Geometry check sheet. Reference: the model listing, model coordinates, mm. A direction names the side the tool comes from. Coordinates: 2 decimals unless noted, no trailing zeros. Loops run counter-clockwise (first coordinate to the right, second up) from the corner with the lowest first, then second, coordinate; pieces in that order, holes last.
Autodesk Inventor part; units mm, degrees
ref_plane "YZ Plane" through (0, 0, 0) normal (1, 0, 0) x (0, 1, 0)
ref_plane "XZ Plane" through (0, 0, 0) normal (0, 1, 0) x (-1, 0, 0)
ref_plane "XY Plane" through (0, 0, 0) normal (0, 0, 1) x (1, 0, 0)
sketch "Sketch1" plane through (0, 0, 0) normal (0, 0, 1) x (1, 0, 0)
  line L0 (0, 0) -> (25.4, 0)
  line L1 (25.4, 0) -> (25.4, 50.8)
  line L2 (25.4, 50.8) -> (0, 50.8)
  line L3 (0, 50.8) -> (0, 0)
  dimension "d0" = 25.4
  dimension "d1" = 50.8
extrude "Extrusion1" add sketch "Sketch1" along normal blind 254
shell "Shell1" thickness 2.54 removed faces 2 at (8.4667, 33.8667, 0) at (8.4667, 33.8667, 254)
sketch "Sketch2" plane through (0, 50.8, 0) normal (0, 1, 0) x (1, 0, 0)
  line L0 (25.4, 0) -> (0, 0)
  line L1 (0, 0) -> (0, -254)
  point P0 (12.7, -12.7)
  point P1 (12.7, -38.1)
  point P2 (12.7, -63.5)
  point P3 (12.7, -88.9)
  point P4 (12.7, -114.3)
  point P5 (12.7, -139.7)
  point P6 (12.7, -165.1)
  point P7 (12.7, -190.5)
  point P8 (12.7, -215.9)
  point P9 (12.7, -241.3)
  point P10 (12.7, -266.7)
  point P11 (12.7, -292.1)
  point P12 (12.7, -317.5)
  point P13 (12.7, -342.9)
  point P14 (12.7, -368.3)
  point P15 (12.7, -393.7)
  point P16 (12.7, -419.1)
  point P17 (12.7, -444.5)
  point P18 (12.7, -469.9)
  point P19 (12.7, -495.3)
  point P20 (12.7, -520.7)
  point P21 (12.7, -546.1)
  point P22 (12.7, -571.5)
  point P23 (12.7, -596.9)
  point P24 (12.7, -622.3)
  point P25 (12.7, -647.7)
  point P26 (12.7, -673.1)
  point P27 (12.7, -698.5)
  point P28 (12.7, -723.9)
  point P29 (12.7, -749.3)
  point P30 (12.7, -774.7)
  point P31 (12.7, -800.1)
  point P32 (12.7, -825.5)
  point P33 (12.7, -850.9)
  point P34 (12.7, -876.3)
  point P35 (12.7, -901.7)
  point P36 (12.7, -927.1)
  dimension "d5" = 12.7
  dimension "d6" = 12.7
  dimension "d9" = 25.4
hole "Hole1" at (12.7, 50.8, 12.7) at (12.7, 50.8, 38.1) at (12.7, 50.8, 63.5) at (12.7, 50.8, 88.9) at (12.7, 50.8, 114.3) at (12.7, 50.8, 139.7) at (12.7, 50.8, 165.1) at (12.7, 50.8, 190.5) at (12.7, 50.8, 215.9) at (12.7, 50.8, 241.3) at (12.7, 50.8, 266.7) at (12.7, 50.8, 292.1) at (12.7, 50.8, 317.5) at (12.7, 50.8, 342.9) at (12.7, 50.8, 368.3) at (12.7, 50.8, 393.7) at (12.7, 50.8, 419.1) at (12.7, 50.8, 444.5) at (12.7, 50.8, 469.9) at (12.7, 50.8, 495.3) at (12.7, 50.8, 520.7) at (12.7, 50.8, 546.1) at (12.7, 50.8, 571.5) at (12.7, 50.8, 596.9) at (12.7, 50.8, 622.3) at (12.7, 50.8, 647.7) at (12.7, 50.8, 673.1) at (12.7, 50.8, 698.5) at (12.7, 50.8, 723.9) at (12.7, 50.8, 749.3) at (12.7, 50.8, 774.7) at (12.7, 50.8, 800.1) at (12.7, 50.8, 825.5) at (12.7, 50.8, 850.9) at (12.7, 50.8, 876.3) at (12.7, 50.8, 901.7) direction (0, -1, 0) diameter 2.54 depth 50.8 tip angle 118
properties part number "Support Pivs cross 2522" material "Aluminum 6061"
1) Access from +Z, -Z, +X, -X, +Y, -Y to the whole of each face (thin tool, end or side, straight path). Record for faces 5 (the flat face through (2.54, 26, 125)), 6 (the flat face through (2, 27, 254)).
Data:
face 5: +Z, -Z
face 6: +Z, +X, -X, +Y, -Y
2) Section check C-C on x = 18.75. Record the cut outline in (y, z).
Data:
outline: (0, 0) - (2.54, 0) - (2.54, 254) - (0, 254) - close; (48.26, 0) - (50.8, 0) - (50.8, 254) - (48.26, 254) - close
3) Section check B-B on z = 197.5. Record the cut outline in (x, y), and give its area (3 significant figures).
Data:
outline: (0, 0) - (25.4, 0) - (25.4, 50.8) - (0, 50.8) - close; hole (2.54, 2.54) - (22.86, 2.54) - (22.86, 48.26) - (2.54, 48.26) - close
area: 361 mm2
4) Material ranges on probe 1 along X at (y, z) = (14.5, 161); probe 2 along Y at (x, z) = (13, 151); probe 3 along X at (y, z) = (49.65, 190.5), recorded low to high.
Data:
probe 1: x = 0 to 2.54, 22.86 to 25.4
probe 2: y = 0 to 2.54, 48.26 to 50.8
probe 3: x = 0 to 11.43, 13.97 to 25.4
5) Mould release check, pull along Y, two halves, no side actions. Record for faces 1 (the flat face through (0, 26, 125)), 2 (the flat face through (13, 50.8, 125)), 3 (the flat face through (13, 0, 125)), 4 (the flat face through (22.86, 25, 125)): +Y half, -Y half, draft (parallel to the pull), parting line (faces both ways), or undercut.
Data:
face 1: draft
face 2: +Y half
face 3: -Y half
face 4: undercut
6) Section check A-A on y = 21. Record the cut outline in (x, z), and give its area (3 significant figures).
Data:
outline: (0, 0) - (2.54, 0) - (2.54, 254) - (0, 254) - close; (22.86, 0) - (25.4, 0) - (25.4, 254) - (22.86, 254) - close
area: 1,290 mm2
